Read the model definition and answer for the solid it produces. Units are mm, in the model's axes. A direction names the side the tool comes from. Give positions to 0.01 mm unless a question says otherwise; leave off trailing zeros. Order: outer loops, then holes, each group sorted by start corner. A loop starts at its lowest first (then second) coordinate and runs counter-clockwise, first axis right, second up.
Item 1: A cutting plane is placed at A-A (y = 7). Write down the section's boundary in (x, z), plus the area to 3 significant figures.
Item 2: Given pin 1 Ø5 at (x, z) = (-102.26, 58.69) entering from -Y; pin 2 Ø2.5 at (x, z) = (-102.66, 218.69) entering from -Y, each flat-ended and moving along its own axis, determine where each tip first touches the part or whether it passes through.
Item 3: Which of the six approach directions +Z, -Z, +X, -X, +Y, -Y give full straight-line access (tool end or side, diameter ignored) to faces 5 (the face through (-91.227, -23, 120)), 6 (the face through (-90.601, -10.576, 162.91)), 7 (the face through (-115, -12, 237.3))?
Item 4: Find the intervals of material crossed by line 1 along X through (y, z) = (-28, 101); line 2 along Y through (x, z) = (-92, 17), in increasing order.
Item 5: The mould has two halves that part along Y. Classify faces 1 (the face through (-103, -37.279, 117)), 2 (the face through (-90.601, -10.324, 183.261)), 3 (the face through (-115.357, -18, 117)), 4 (the face through (-114.731, -10.324, 131.269)): +Y half, -Y half, draft (parallel to the pull), parting line (faces both ways), or undercut.
Item 6: A cutting plane is placed at D-D (y = -15). State how many separate pieces and enclosed holes the cut face has, plus the area to 3 significant figures.
Item 7: A cutting plane is placed at C-C (z = 51). Write down the section's boundary in (x, y), plus the area to 3 significant figures.
Item 8: A cutting plane is placed at B-B (x = -96.5). Write down the section's boundary in (y, z), plus the area to 3 significant figures.
from build123d import *

# Parameters (mm, degrees)
SKETCH1_W           = 25.4
SKETCH1_H           = 50.8
SKETCH1_W_2         = 22.86
SKETCH1_H_2         = 48.26
BOSS_EXTRUDE1_DEPTH = 237.2995
CUT_EXTRUDE1_DEPTH  = 242.549111961
FILLET1_R           = 3
MIRROR1_START       = -91.227065342
MIRROR1_DEPTH       = 1.27
SKETCH6_R           = 1.5
CUT_EXTRUDE2_DEPTH  = 269.69861411


# Read off the part's stored shape, not the designer's step: Mirror1
with BuildPart() as part:
    # Sketch1 → Boss-Extrude1 (new body)
    with BuildSketch(Plane.XY):
        with Locations((-102.657065342, -11.879495554)):
            Rectangle(SKETCH1_W, SKETCH1_H)
        with Locations((-102.657065342, -11.879495554)):
            Rectangle(SKETCH1_W_2, SKETCH1_H_2, mode=Mode.SUBTRACT)
    extrude(amount=BOSS_EXTRUDE1_DEPTH)

    # Sketch5 → Cut-Extrude1 (cut, through all)
    with BuildSketch(Plane.ZY.offset(115.357065342)):
        Polygon((59.65825413, -27.279495554), (37.1624375, -1.771064943), (14.66662087, -27.279495554), align=None)
        Polygon((68.99149587, -27.279495554), (92.653967718, -0.448172595), (116.316439565, -27.279495554), align=None)
        Polygon((98.487243806, 3.520504446), (143.478877065, 3.520504446), (120.983060435, -21.987926165), align=None)
        Polygon((125.649681306, -27.279495554), (146.978842718, -3.09395729), (168.30800413, -27.279495554), align=None)
        Polygon((150.47880837, 3.520504446), (195.47044163, 3.520504446), (172.974625, -21.987926165), align=None)
        Polygon((177.64124587, -27.279495554), (200.1370625, -1.771064943), (222.63287913, -27.279495554), align=None)
        Polygon((41.82905837, 3.520504446), (86.82069163, 3.520504446), (64.324875, -21.987926165), align=None)
    extrude(amount=-CUT_EXTRUDE1_DEPTH, mode=Mode.SUBTRACT)

    # Fillet1
    fillet1_edges = [part.edges().sort_by_distance(p)[0] for p in [
        (-114.722065342, 3.520504446, 41.82905837),
        (-114.722065342, 3.520504446, 86.82069163),
        (-114.722065342, -21.987926165, 64.324875),
        (-114.722065342, -1.771064943, 37.1624375),
        (-114.722065342, -27.279495554, 59.65825413),
        (-114.722065342, -27.279495554, 14.66662087),
        (-114.722065342, -27.279495554, 125.649681306),
        (-114.722065342, -3.09395729, 146.978842718),
        (-114.722065342, -27.279495554, 168.30800413),
        (-114.722065342, 3.520504446, 150.47880837),
        (-114.722065342, 3.520504446, 195.47044163),
        (-114.722065342, -21.987926165, 172.974625),
        (-114.722065342, -27.279495554, 68.99149587),
        (-114.722065342, -0.448172595, 92.653967718),
        (-114.722065342, -27.279495554, 116.316439565),
        (-114.722065342, 3.520504446, 98.487243806),
        (-114.722065342, 3.520504446, 143.478877065),
        (-114.722065342, -21.987926165, 120.983060435),
        (-114.722065342, -27.279495554, 177.64124587),
        (-114.722065342, -1.771064943, 200.1370625),
        (-114.722065342, -27.279495554, 222.63287913),
    ]]
    fillet(fillet1_edges, radius=FILLET1_R)

    # Mirror1 outline → Mirror1 (add)
    with BuildSketch(Plane.YZ.offset(MIRROR1_START)):
        with BuildLine():
            ThreePointArc((-19.436583706, 170.724602919), (-20.45229526, 172.974625), (-19.436583706, 175.224647081))
            Line((-19.436583706, 175.224647081), (-21.987926165, 172.974625))
            Line((-21.987926165, 172.974625), (-19.436583706, 170.724602919))
        make_face()
        with BuildLine():
            Line((3.520504446, 195.47044163), (-1.463784, 191.074811))
            ThreePointArc((-1.463784, 191.074811), (1.754833143, 191.559095535), (3.520504446, 188.824788919))
            Line((3.520504446, 188.824788919), (3.520504446, 195.47044163))
        make_face()
        with BuildLine():
            ThreePointArc((3.520504446, 157.124461081), (1.754833143, 154.390154465), (-1.463784, 154.874439))
            Line((-1.463784, 154.874439), (3.520504446, 150.47880837))
            Line((3.520504446, 150.47880837), (3.520504446, 157.124461081))
        make_face()
        with BuildLine():
            Line((3.520504446, 143.478877065), (-1.463784, 139.083246435))
            ThreePointArc((-1.463784, 139.083246435), (1.754833143, 139.56753097), (3.520504446, 136.833224354))
            Line((3.520504446, 136.833224354), (3.520504446, 143.478877065))
        make_face()
        with BuildLine():
            ThreePointArc((-19.436583706, 118.733038355), (-20.45229526, 120.983060435), (-19.436583706, 123.233082516))
            Line((-19.436583706, 123.233082516), (-21.987926165, 120.983060435))
            Line((-21.987926165, 120.983060435), (-19.436583706, 118.733038355))
        make_face()
        with BuildLine():
            Line((3.520504446, 98.487243806), (3.520504446, 105.132896516))
            ThreePointArc((3.520504446, 105.132896516), (1.754833143, 102.3985899), (-1.463784, 102.882874435))
            Line((-1.463784, 102.882874435), (3.520504446, 98.487243806))
        make_face()
        with BuildLine():
            Line((-27.279495554, 125.649681306), (-22.295207108, 130.045311935))
            ThreePointArc((-22.295207108, 130.045311935), (-25.513824251, 129.5610274), (-27.279495554, 132.295334016))
            Line((-27.279495554, 132.295334016), (-27.279495554, 125.649681306))
        make_face()
        with BuildLine():
            ThreePointArc((-5.645299749, 149.228864798), (-4.629588195, 146.978842718), (-5.645299749, 144.728820637))
            Line((-5.645299749, 144.728820637), (-3.09395729, 146.978842718))
            Line((-3.09395729, 146.978842718), (-5.645299749, 149.228864798))
        make_face()
        with BuildLine():
            Line((-27.279495554, 168.30800413), (-27.279495554, 161.662351419))
            ThreePointArc((-27.279495554, 161.662351419), (-25.513824251, 164.396658035), (-22.295207108, 163.9123735))
            Line((-22.295207108, 163.9123735), (-27.279495554, 168.30800413))
        make_face()
        with BuildLine():
            Line((-27.279495554, 177.64124587), (-22.295207108, 182.0368765))
            ThreePointArc((-22.295207108, 182.0368765), (-25.513824251, 181.552591965), (-27.279495554, 184.286898581))
            Line((-27.279495554, 184.286898581), (-27.279495554, 177.64124587))
        make_face()
        with BuildLine():
            ThreePointArc((-4.322407402, 202.387084581), (-3.306695848, 200.1370625), (-4.322407402, 197.887040419))
            Line((-4.322407402, 197.887040419), (-1.771064943, 200.1370625))
            Line((-1.771064943, 200.1370625), (-4.322407402, 202.387084581))
        make_face()
        with BuildLine():
            Line((-27.279495554, 222.63287913), (-27.279495554, 215.987226419))
            ThreePointArc((-27.279495554, 215.987226419), (-25.513824251, 218.721533035), (-22.295207108, 218.2372485))
            Line((-22.295207108, 218.2372485), (-27.279495554, 222.63287913))
        make_face()
        with BuildLine():
            Line((-27.279495554, 116.316439565), (-27.279495554, 109.670786854))
            ThreePointArc((-27.279495554, 109.670786854), (-25.513824251, 112.40509347), (-22.295207108, 111.920808935))
            Line((-22.295207108, 111.920808935), (-27.279495554, 116.316439565))
        make_face()
        with BuildLine():
            ThreePointArc((-22.295207108, 73.3871265), (-25.513824251, 72.902841965), (-27.279495554, 75.637148581))
            Line((-27.279495554, 75.637148581), (-27.279495554, 68.99149587))
            Line((-27.279495554, 68.99149587), (-22.295207108, 73.3871265))
        make_face()
        with BuildLine():
            Line((-0.448172595, 92.653967718), (-2.999515054, 94.903989798))
            ThreePointArc((-2.999515054, 94.903989798), (-1.9838035, 92.653967717), (-2.999515054, 90.403945637))
            Line((-2.999515054, 90.403945637), (-0.448172595, 92.653967718))
        make_face()
        with BuildLine():
            Line((3.520504446, 86.82069163), (-1.463784, 82.425061))
            ThreePointArc((-1.463784, 82.425061), (1.754833143, 82.909345535), (3.520504446, 80.175038919))
            Line((3.520504446, 80.175038919), (3.520504446, 86.82069163))
        make_face()
        with BuildLine():
            ThreePointArc((-19.436583706, 62.074852919), (-20.45229526, 64.324875), (-19.436583706, 66.574897081))
            Line((-19.436583706, 66.574897081), (-21.987926165, 64.324875))
            Line((-21.987926165, 64.324875), (-19.436583706, 62.074852919))
        make_face()
        with BuildLine():
            Line((3.520504446, 41.82905837), (3.520504446, 48.474711081))
            ThreePointArc((3.520504446, 48.474711081), (1.754833143, 45.740404465), (-1.463784, 46.224689))
            Line((-1.463784, 46.224689), (3.520504446, 41.82905837))
        make_face()
        with BuildLine():
            ThreePointArc((-27.279495554, 53.012601419), (-25.513824251, 55.746908035), (-22.295207108, 55.2626235))
            Line((-22.295207108, 55.2626235), (-27.279495554, 59.65825413))
            Line((-27.279495554, 59.65825413), (-27.279495554, 53.012601419))
        make_face()
        with BuildLine():
            Line((-1.771064943, 37.1624375), (-4.322407402, 39.412459581))
            ThreePointArc((-4.322407402, 39.412459581), (-3.306695848, 37.1624375), (-4.322407402, 34.912415419))
            Line((-4.322407402, 34.912415419), (-1.771064943, 37.1624375))
        make_face()
        with BuildLine():
            ThreePointArc((-22.295207108, 19.0622515), (-25.513824251, 18.577966965), (-27.279495554, 21.312273581))
            Line((-27.279495554, 21.312273581), (-27.279495554, 14.66662087))
            Line((-27.279495554, 14.66662087), (-22.295207108, 19.0622515))
        make_face()
    extrude(amount=MIRROR1_DEPTH)

    # Sketch6 → Cut-Extrude2 (cut, through all)
    with BuildSketch(Plane(origin=(0, 13.520504446, 0), x_dir=(1, 0, 0), z_dir=(0, 1, 0))):
        with Locations(Location((-102.657065342, -138.6915017, 0), (0, 0, 270))):
            Circle(SKETCH6_R)
        with Locations(Location((-102.657065342, -178.6915017, 0), (0, 0, 270))):
            Circle(SKETCH6_R)
        with Locations(Location((-102.657065342, -218.6915017, 0), (0, 0, 270))):
            Circle(SKETCH6_R)
        with Locations(Location((-102.001257873, -18.693437093, 0), (0, 0, 90))):
            Circle(SKETCH6_R)
        with Locations(Location((-102.263580578, -58.692576918, 0), (0, 0, 90))):
            Circle(SKETCH6_R)
        with Locations(Location((-102.525903284, -98.691716744, 0), (0, 0, 90))):
            Circle(SKETCH6_R)
    extrude(amount=-CUT_EXTRUDE2_DEPTH, mode=Mode.SUBTRACT)


solid = part.part
Response values:
1. outline: (-115.36, 0) - (-114.09, 0) - (-114.09, 237.3) - (-115.36, 237.3) - close; (-91.23, 0) - (-89.96, 0) - (-89.96, 237.3) - (-91.23, 237.3) - close
1. area: 603 mm2
2. pin 1: stops at y = -37.28
2. pin 2: passes through
3. face 5: +Z, -Z
3. face 6: +X, -X
3. face 7: +Z, +X, -X, +Y, -Y
4. line 1: x = -115.36 to -114.09, -91.23 to -89.96
4. line 2: y = -37.28 to -36.01, 12.25 to 13.52
5. face 1: -Y half
5. face 2: undercut
5. face 3: draft
5. face 4: undercut
6. separate pieces: 16
6. enclosed holes: 0
6. area: 272 mm2
7. outline: (-115.36, -37.28) - (-89.96, -37.28) - (-89.96, -27.28) - (-91.23, -27.28) - (-91.23, -36.01) - (-114.09, -36.01) - (-114.09, -27.28) - (-115.36, -27.28) - close; (-115.36, -17.46) - (-114.09, -17.46) - (-114.09, -6.88) - (-115.36, -6.88) - close; (-115.36, 3.52) - (-114.09, 3.52) - (-114.09, 12.25) - (-91.23, 12.25) - (-91.23, 3.52) - (-89.96, 3.52) - (-89.96, 13.52) - (-115.36, 13.52) - close; (-91.23, -17.46) - (-89.96, -17.46) - (-89.96, -6.88) - (-91.23, -6.88) - close
7. area: 136 mm2
8. outline: (-37.28, 0) - (-36.01, 0) - (-36.01, 237.3) - (-37.28, 237.3) - close; (12.25, 0) - (13.52, 0) - (13.52, 237.3) - (12.25, 237.3) - close
8. area: 603 mm2
